Drawing for the job (mm, zero at the part's lowest x, y, z). Round coordinates to 2 decimals unless told otherwise and drop trailing zeros. Write each loop counter-clockwise with the first axis right and the second up, starting at its lowest first coordinate (ties: lowest second). Pieces come first, ordered by that corner, then holes.
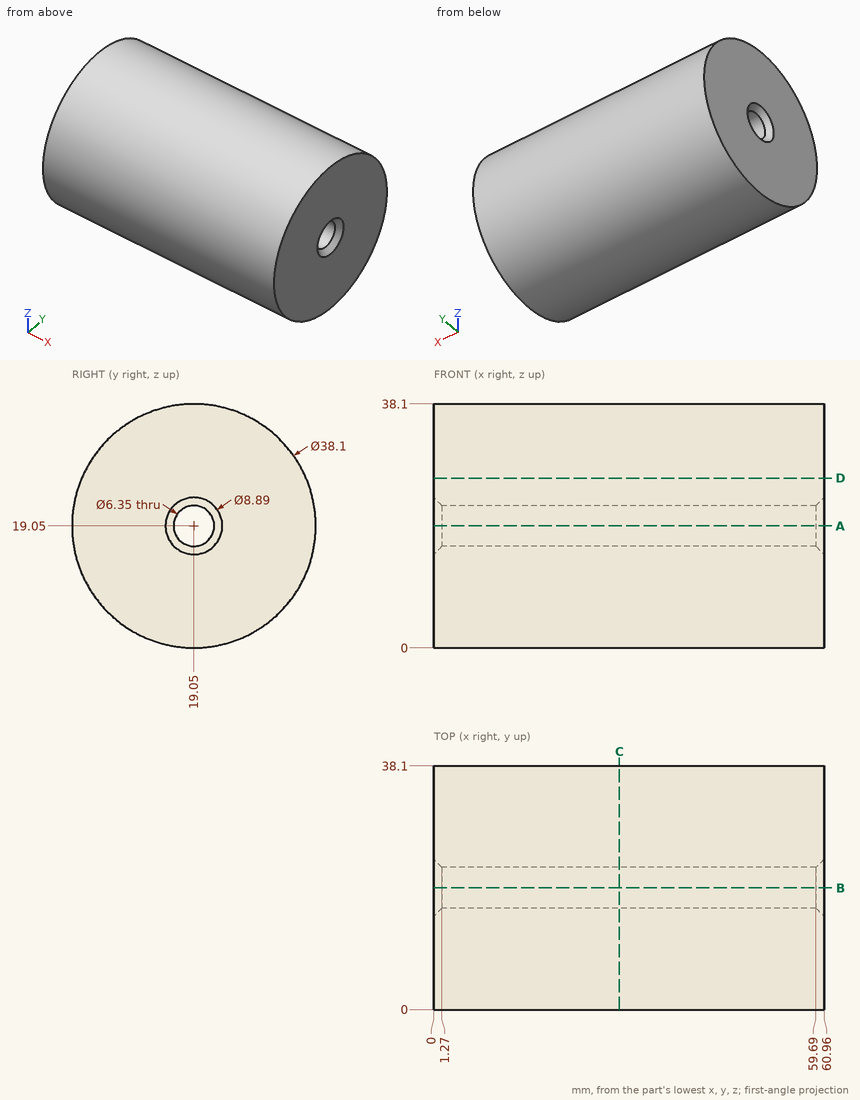
1) Cut at D-D on z = 26.5. List the corners of the cut face in (x, y).
2) Cut at A-A on z = 19.05. List the corners of the cut face in (x, y) (3 decimals), and give its area (3 significant figures).
3) Cut at C-C on x = 29. List the corners of the cut face in (y, z) (3 decimals), and give its area (3 significant figures).
4) Flat gauge pins, fed straight in: pin 1 Ø3 at (x, y) = (52, 18) entering from -Z; pin 2 Ø4 at (x, y) = (35, 28) entering from -Z; pin 3 Ø8 at (x, z) = (52.5, 4.5) entering from -Y. Where does each tip first touch, or does it go through?
5) Wall check: probe 1 along Z at (x, y) = (45.5, 19.05) (3 decimals); probe 2 along Y at (x, z) = (15, 19); probe 3 along Z at (x, y) = (42.5, 17.5). Give the ranges that are in metal, low to high.
Result sheet:
1. outline: (0, 1.52) - (60.96, 1.52) - (60.96, 36.58) - (0, 36.58) - close
2. outline: (0, 0) - (60.96, 0) - (60.96, 14.605) - (59.69, 15.875) - (1.27, 15.875) - (0, 14.605) - close; (0, 23.495) - (1.27, 22.225) - (59.69, 22.225) - (60.96, 23.495) - (60.96, 38.1) - (0, 38.1) - close
2. area: 1,930 mm2
3. outline: circle Ø38.1 at (19.05, 19.05); hole circle Ø6.35 at (19.05, 19.05)
3. area: 1,110 mm2
4. pin 1: stops at z = 0
4. pin 2: stops at z = 1.31
4. pin 3: stops at y = 3.19
5. probe 1: z = 0 to 15.875, 22.225 to 38.1
5. probe 2: y = 0 to 15.88, 22.22 to 38.1
5. probe 3: z = 0.06 to 16.28, 21.82 to 38.04
